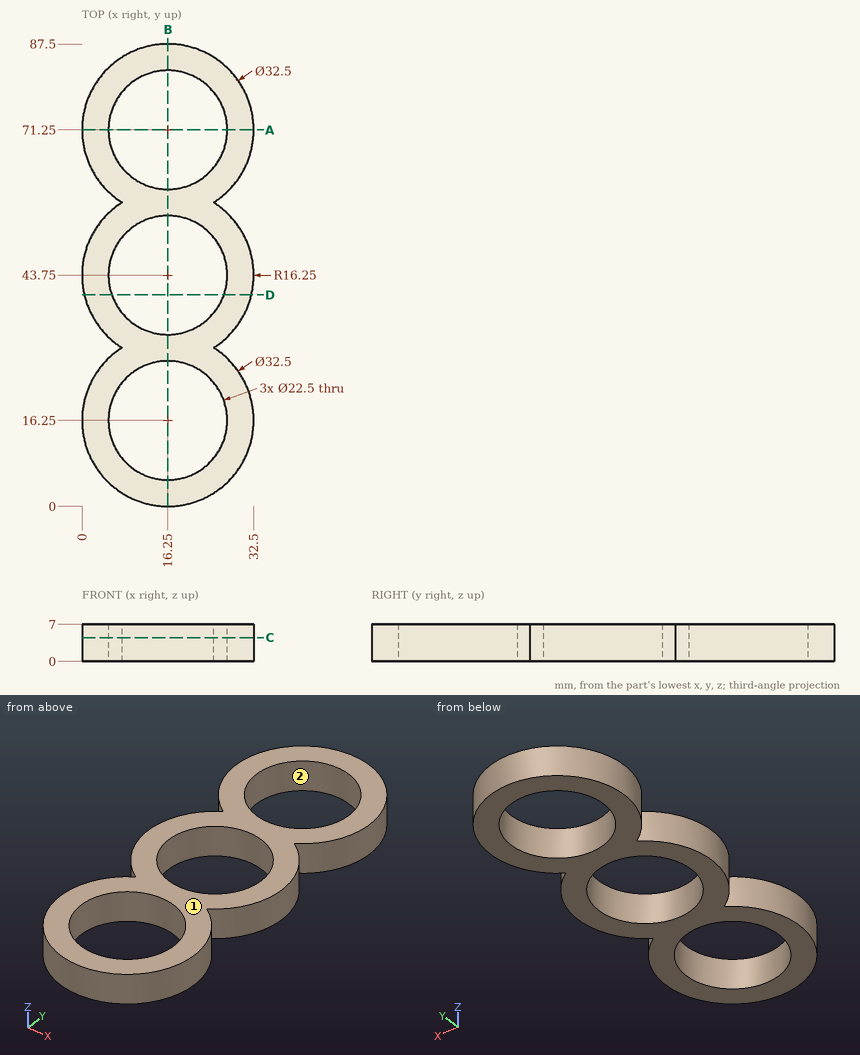
Check sheet for the drawn part. Datum: minimum x, y, z corner. Units: mm. Round coordinates to 2 decimals unless told otherwise and drop trailing zeros. Order: outer loops, then holes, each group sorted by start corner. A loop starts at its lowest first (then second) coordinate and runs counter-clockwise, first axis right, second up. Notation, with made-up numbers: M 37.5,-19.75 L 71.5,-19.75 A10 ccw 71.5,-9.75 Z; hole C 29,2 d7. An arc over 180 degrees is marked long. Answer in a Markdown table with one row per item.
(1) Material ranges on line 1 along X through (y, z) = (16.5, 4.75); line 2 along Y through (x, z) = (4, 4.5); line 3 along Y through (x, z) = (20, 2.5), recorded low to high. Write a range as from..to.
Findings:
| item | result |
|---|---|
| line 1 | x = 0..5, 27.5..32.5 |
| line 2 | y = 5.57..26.93, 33.07..54.43, 60.57..81.93 |
| line 3 | y = 0.44..5.64, 26.86..33.14, 54.36..60.64, 81.86..87.06 |
(2) Section check B-B on x = 16.25. Record the boundary of the cut face in (y, z), plus the area to 3 significant figures.
Findings:
| item | result |
|---|---|
| outline | M 0,0 L 5,0 L 5,7 L 0,7 Z; M 27.5,0 L 32.5,0 L 32.5,7 L 27.5,7 Z; M 55,0 L 60,0 L 60,7 L 55,7 Z; M 82.5,0 L 87.5,0 L 87.5,7 L 82.5,7 Z |
| area | 140 mm^2 |
(3) Draft check along X on the marked faces 1 and 2. Enter one of: +X half, -X half, draft (parallel to the pull), parting line (faces both ways), or undercut.
Findings:
| item | result |
|---|---|
| face 1 | draft |
| face 2 | undercut |
(4) Section check A-A on y = 71.25. Record the boundary of the cut face in (x, z).
Findings:
| item | result |
|---|---|
| outline | M 0,0 L 5,0 L 5,7 L 0,7 Z; M 27.5,0 L 32.5,0 L 32.5,7 L 27.5,7 Z |
(5) Section check C-C on z = 4.5. Record the boundary of the cut face in (x, y), plus the area to 3 significant figures.
Findings:
| item | result |
|---|---|
| outline | M 7.59,30 A16.25 ccw long 24.91,30 A16.25 ccw 24.91,57.5 A16.25 ccw long 7.59,57.5 A16.25 ccw Z; hole C 16.25,16.25 d22.5; hole C 16.25,43.75 d22.5; hole C 16.25,71.25 d22.5 |
| area | 1,180 mm^2 |
(6) Section check D-D on y = 40. Record the boundary of the cut face in (x, z), plus the area to 3 significant figures.
Findings:
| item | result |
|---|---|
| outline | M 0.44,0 L 5.64,0 L 5.64,7 L 0.44,7 Z; M 26.86,0 L 32.06,0 L 32.06,7 L 26.86,7 Z |
| area | 72.9 mm^2 |
